```python
from build123d import *

# Parameters (mm, degrees)
ESQUISSE1_R                                   = 5
BOSS_EXTRU_1_DEPTH                            = 75
ESQUISSE2_R                                   = 3
BOSS_EXTRU_2_DEPTH                            = 10
TROU_POUR_TARAUDAGE_POUR_TROU_TARAUD_M5_D     = 4.2
TROU_POUR_TARAUDAGE_POUR_TROU_TARAUD_M5_DEPTH = 10
TROU_POUR_TARAUDAGE_POUR_TROU_TARAUD_M5_TIP   = 1.2618073
CHANFREIN1_SIZE                               = 0.5


with BuildPart() as part:
    # Esquisse1 → Boss.-Extru.1 (new body)
    with BuildSketch(Plane.XY):
        Circle(ESQUISSE1_R)
    extrude(amount=BOSS_EXTRU_1_DEPTH)

    # Esquisse2 → Boss.-Extru.2 (add)
    with BuildSketch(Plane(origin=(0, 0, 0), x_dir=(-1, 0, 0), z_dir=(0, 0, -1))):
        Circle(ESQUISSE2_R)
    extrude(amount=BOSS_EXTRU_2_DEPTH)

    # Trou pour taraudage pour trou taraudé M51
    with Locations(Plane.XY.offset(75)):
        with Locations((0, 0)):
            Hole(TROU_POUR_TARAUDAGE_POUR_TROU_TARAUD_M5_D / 2, depth=TROU_POUR_TARAUDAGE_POUR_TROU_TARAUD_M5_DEPTH)
            with Locations((0, 0, -(TROU_POUR_TARAUDAGE_POUR_TROU_TARAUD_M5_DEPTH + TROU_POUR_TARAUDAGE_POUR_TROU_TARAUD_M5_TIP / 2))):  # 118° drill point
                Cone(0, TROU_POUR_TARAUDAGE_POUR_TROU_TARAUD_M5_D / 2, TROU_POUR_TARAUDAGE_POUR_TROU_TARAUD_M5_TIP, mode=Mode.SUBTRACT)

    # Chanfrein1
    chanfrein1_edges = [part.edges().sort_by_distance(p)[0] for p in [
        (-5, 0, 0),
        (-5, 0, 75),
        (3, 0, -10),
    ]]
    chamfer(chanfrein1_edges, length=CHANFREIN1_SIZE)


solid = part.part
```
Could you check a few things on this model? Use its own coordinates, in mm. A direction names the side the tool comes from. Round coordinates to 2 decimals unless told otherwise and drop trailing zeros. Write each loop counter-clockwise with the first axis right and the second up, starting at its lowest first coordinate (ties: lowest second). Pieces come first, ordered by that corner, then holes. Notation, with made-up numbers: M 80,13 L 105,13 A15 cw 105,34 Z; hole C 53,-7.5 d1. An arc over 180 degrees is marked long. Write each question's results on one line, items separated by ' | '. Start each with the question number.
1. I'm going to push flat-ended pins straight in: pin 1 Ø1 at (x, z) = (2, 1.5) entering from +Y; pin 2 Ø1 at (x, y) = (2, -2.5) entering from -Z; pin 3 Ø5 at (y, z) = (3, 11) entering from +X. Where does each tip first touch, or does it pass through?
2. On a 3-axis mill with a long thin cutter (end or side, diameter ignored), from which of +Z, -Z, +X, -X, +Y, -Y can I reach the whole of each face in a straight line? I mean faces 4 (the face through (-1.08, -4.88, 36.98)), 5 (the face through (-2.003, 0.631, 69.93)), 6 (the face through (1, -3, 0)). Say none if no direction works.
3. Thinking about a two-plate mould opening in Y: for faces 1 (the face through (0.34, -0.14, 63.96)), 2 (the face through (-2.1, -0.9, 75)), 3 (the face through (3, 0, -5)), which applies, +Y half, -Y half, draft (parallel to the pull), parting line (faces both ways), or undercut?
4. I need wall thicknesses on L1, parallel to Y at x = 0, z = 72.25; L2, parallel to Z at x = -3, y = 2.25; L3, parallel to Y at x = 1.25, z = 70. Which ranges of each line are inside material? Lowest first, please. Write a range as from..to.
5. Imagine slicing it at A-A on z = 31. List the corners of the cut face in (x, y) for me, and give its area (3 significant figures).
Result sheet:
1) pin 1: stops at y = 4.77 | pin 2: stops at z = -9.8 | pin 3: stops at x = 4.97
2) face 4: +Z, -Z | face 5: +Z | face 6: -Z
3) face 1: undercut | face 2: draft | face 3: parting line
4) L1: y = -5..-2.1, 2.1..5 | L2: z = 0..75 | L3: y = -4.84..-1.69, 1.69..4.84
5) outline: C 0,0 d10 | area: 78.5 mm^2
